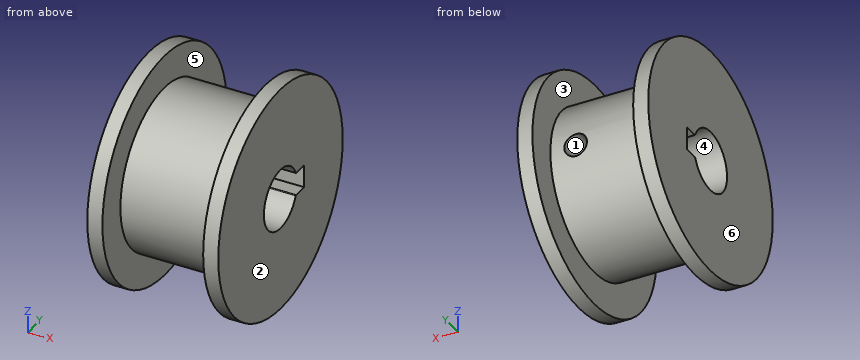
from build123d import *

# Parameters (mm, degrees)
SKETCH1_R               = 16
BOSS_EXTRUDE1_DEPTH     = 20
SKETCH3_R               = 22.5
BOSS_EXTRUDE2_DEPTH     = 3
SKETCH4_R               = 22.5
BOSS_EXTRUDE3_DEPTH     = 3
CUT_EXTRUDE2_DEPTH      = 3
CUT_EXTRUDE2_DEPTH_BACK = 25
SKETCH6_R               = 2.25
CUT_EXTRUDE3_DEPTH      = 10


with BuildPart() as part:
    # Sketch1 → Boss-Extrude1 (new body)
    with BuildSketch(Plane(origin=(0, 0, 0), x_dir=(0, 0, -1), z_dir=(1, 0, 0))):
        Circle(SKETCH1_R)
    extrude(amount=BOSS_EXTRUDE1_DEPTH)

    # Sketch3 → Boss-Extrude2 (add)
    with BuildSketch(Plane(origin=(20, 0, 0), x_dir=(0, 0, -1), z_dir=(1, 0, 0))):
        Circle(SKETCH3_R)
    extrude(amount=BOSS_EXTRUDE2_DEPTH)

    # Sketch4 → Boss-Extrude3 (add)
    with BuildSketch(Plane.ZY):
        Circle(SKETCH4_R)
    extrude(amount=BOSS_EXTRUDE3_DEPTH)

    # Sketch2 → Cut-Extrude2 (cut, two sides)
    with BuildSketch(Plane(origin=(20, 0, 0), x_dir=(0, 0, -1), z_dir=(1, 0, 0))) as cut_extrude2_sk:
        with BuildLine():
            Line((-2.25, 8.562148865), (2.25, 8.562148865))
            Line((2.25, 8.562148865), (2.25, 5.695392875))
            ThreePointArc((2.25, 5.695392875), (2.282957413, 5.585407539), (2.370967742, 5.511670524))
            ThreePointArc((2.370967742, 5.511670524), (0, -6), (-2.370967742, 5.511670524))
            ThreePointArc((-2.370967742, 5.511670524), (-2.282957413, 5.585407539), (-2.25, 5.695392875))
            Line((-2.25, 5.695392875), (-2.25, 8.562148865))
        make_face()
    extrude(amount=CUT_EXTRUDE2_DEPTH, mode=Mode.SUBTRACT)
    extrude(cut_extrude2_sk.sketch, amount=-CUT_EXTRUDE2_DEPTH_BACK, mode=Mode.SUBTRACT)

    # Sketch6 → Cut-Extrude3 (cut)
    with BuildSketch(Plane.XZ.offset(-8.562148865)):
        with Locations((15, 0)):
            Circle(SKETCH6_R)
    extrude(amount=-CUT_EXTRUDE3_DEPTH, mode=Mode.SUBTRACT)


solid = part.part
Geometry: final body of the model. Coordinates: model frame, mm. Face numbers are marked on the shaded views. A direction names the side the tool comes from. Round coordinates to 2 decimals unless told otherwise and drop trailing zeros. Loops run counter-clockwise (first coordinate to the right, second up) from the corner with the lowest first, then second, coordinate; pieces in that order, holes last.
Q1. Pull-direction query (X, two-part tool) for the marked faces 4, 5 and 6; classes: released by +X, released by -X, zero draft, split by the parting line, or undercut.
Q2. Section A-A on z = 0. Return loops of the section in (x, y).
Q3. Section D-D on z = -17. Return loops of the section in (x, y).
Q4. Access query for the marked faces 1, 2 and 3. Directions: +Z, -Z, +X, -X, +Y, -Y. A direction counts if a zero-diameter tool reaches every point of the face in a straight line with its end or side. Return the directions, or none.
Q5. Material intervals for L1, parallel to Y at x = 2.75, z = 0; L2, parallel to X at y = 11, z = 0; L3, parallel to X at y = 19, z = 12, sorted ascending.
Q6. Pin query (flat end, axial travel): P1, Ø4, axis at x = 4, y = 11.5, coming from the -Z side; P2, Ø0.9, axis at x = 5.5, y = 6.5, coming from the -Z side; P3, Ø1, axis at x = 4.5, z = -1.5, coming from the +Y side. Return the tip coordinate at first contact, or that it passes through.
Q7. Section B-B on y = 0. Return loops of the section in (x, z), plus the area to 3 significant figures.
Q8. Section C-C on x = 18.5. Return loops of the section in (y, z), plus the area to 3 significant figures.
Evaluation:
1. face 4: zero draft
1. face 5: undercut
1. face 6: released by -X
2. outline: (-3, -22.5) - (0, -22.5) - (0, -16) - (20, -16) - (20, -22.5) - (23, -22.5) - (23, -6) - (-3, -6) - close; (-3, 8.56) - (12.75, 8.56) - (12.75, 16) - (0, 16) - (0, 22.5) - (-3, 22.5) - close; (17.25, 8.56) - (23, 8.56) - (23, 22.5) - (20, 22.5) - (20, 16) - (17.25, 16) - close
3. outline: (-3, -14.74) - (0, -14.74) - (0, 14.74) - (-3, 14.74) - close; (20, -14.74) - (23, -14.74) - (23, 14.74) - (20, 14.74) - close
4. face 1: +Y
4. face 2: +Z, -Z, +X, +Y, -Y
4. face 3: none
5. L1: y = -16 to -6, 8.56 to 16
5. L2: x = -3 to 12.75, 17.25 to 23
5. L3: x = -3 to 0, 20 to 23
6. P1: stops at z = -12.87
6. P2: stops at z = -14.81
6. P3: stops at y = 15.97
7. outline: (-3, -22.5) - (0, -22.5) - (0, -16) - (20, -16) - (20, -22.5) - (23, -22.5) - (23, -6) - (-3, -6) - close; (-3, 6) - (23, 6) - (23, 22.5) - (20, 22.5) - (20, 16) - (0, 16) - (0, 22.5) - (-3, 22.5) - close
7. area: 598 mm2
8. outline: circle Ø32 at (0, 0); hole (5.51, -2.37) arc R0.2 cw to (5.7, -2.25) - (8.56, -2.25) - (8.56, 2.25) - (5.7, 2.25) arc R0.2 cw to (5.51, 2.37) arc R6 ccw (long way) to start
8. area: 679 mm2
